```python
from build123d import *

# Parameters (mm, degrees)
BOSS_EXTRUDE1_DEPTH = 6
CHAMFER1_SIZE       = 1
SKETCH2_R           = 1.5
BOSS_EXTRUDE2_DEPTH = 0.7
CHAMFER2_SIZE       = 1
FILLET1_R           = 0.5
BOSS_EXTRUDE3_DEPTH = 1
BOSS_EXTRUDE4_START = 6
BOSS_EXTRUDE4_DEPTH = 1


with BuildPart() as part:
    # Sketch1 → Boss-Extrude1 (new body)
    with BuildSketch(Plane.XY):
        with BuildLine():
            ThreePointArc((0.3, -8), (-0.712809438, -8.999917956), (-1.699671837, -7.974383226))
            Line((-1.699671837, -7.974383226), (-0.822800703, -2.420866047))
            Line((-0.822800703, -2.420866047), (-1.647054908, -1.729905435))
            Line((-1.647054908, -1.729905435), (-1.454328442, -1.5))
            Line((-1.454328442, -1.5), (-0.5, -2.3))
            Line((-0.5, -2.3), (-1.4, -8))
            ThreePointArc((-1.4, -8), (-0.7, -8.7), (0, -8))
            Line((0, -8), (0, 0))
            Line((0, 0), (0.3, 0))
            Line((0.3, 0), (0.3, -8))
        make_face()
    extrude(amount=BOSS_EXTRUDE1_DEPTH)

    # Chamfer1
    chamfer1_edges = [part.edges().sort_by_distance(p)[0] for p in [
        (-1.550691675, -1.614952718, 0),
        (-1.550691675, -1.614952718, 6),
    ]]
    chamfer(chamfer1_edges, length=CHAMFER1_SIZE)

    # Sketch2 → Boss-Extrude2 (add)
    with BuildSketch(Plane(origin=(0.3, 0, 0), x_dir=(0, 0, -1), z_dir=(1, 0, 0))):
        with Locations((-3, -4.3)):
            Circle(SKETCH2_R)
    extrude(amount=BOSS_EXTRUDE2_DEPTH)

    # Chamfer2
    # the kernel refuses this chamfer: 1 mm, written as the material it adds along each edge
    with BuildSketch(Plane(origin=(0.3, -4.3, 3), x_dir=(0, 0, -1), z_dir=(0, -1, 0))) as chamfer2_piece_1_section:
        Polygon((1.5 + CHAMFER2_SIZE, 0), (1.5, CHAMFER2_SIZE), (1.5, 0), align=None)
    chamfer2_piece_1 = revolve(axis=Axis((0.3, -4.3, 3), (1, 0, 0)), mode=Mode.PRIVATE)
    chamfer2_piece_1 = split(chamfer2_piece_1, bisect_by=Plane(origin=(1, -4.3, 5.151462954), z_dir=(-1, 0, 0)), keep=Keep.TOP, mode=Mode.PRIVATE)
    add(chamfer2_piece_1)

    # Fillet1
    fillet1_edges = [part.edges().sort_by_distance(p)[0] for p in [
        (0.3, -4.3, 5.5),
        (1, -4.3, 4.8),
    ]]
    fillet(fillet1_edges, radius=FILLET1_R)

    # Sketch1<3> → Boss-Extrude3 (add)
    with BuildSketch(Plane.XY):
        Polygon((-0.878934414, -4.699917956), (-0.962606384, -5.229840435), (-0.621188888, -5.961100292), (-0.349357155, -5.83418493), align=None)
    extrude(amount=BOSS_EXTRUDE3_DEPTH)

    # Sketch1<4> → Boss-Extrude4 (add)
    with BuildSketch(Plane.XY.offset(BOSS_EXTRUDE4_START)):
        Polygon((-0.878934414, -4.699917956), (-0.962606384, -5.229840435), (-0.621188888, -5.961100292), (-0.349357155, -5.83418493), align=None)
    extrude(amount=-BOSS_EXTRUDE4_DEPTH)


solid = part.part
```
Source: CAD feature listing. Evaluate the final solid. Frame: model axes, mm. A direction names the side the tool comes from. Coordinates: 2 decimals unless noted, no trailing zeros. Write each loop counter-clockwise with the first axis right and the second up, starting at its lowest first coordinate (ties: lowest second). Pieces come first, ordered by that corner, then holes. Notation, with made-up numbers: M 16,-39 L 47,-39 A7 cw 47,-33 Z; hole C 0,31 d1. An arc over 180 degrees is marked long. Answer as a JSON object with one key per item and string values.
1. Access query for faces 1 (the flat face through (0, -4, 3)), 2 (the flat face through (1, -4, 3)), 3 (the flat face through (-0.6, -5.3, 5.5)), 4 (the flat face through (-1.267, -5.236, 2.958)). Directions: +Z, -Z, +X, -X, +Y, -Y. A direction counts if a zero-diameter tool reaches every point of the face in a straight line with its end or side. Return the directions, or none.
Evaluation:
{"face 1": "+Z, -Z, +Y", "face 2": "+Z, -Z, +X, +Y, -Y", "face 3": "+Z, -Z", "face 4": "+Z, -Z, -X"}
2. Cut plane C-C on y = -1.25. Output: boundary loops of the cut face in (x, z).
Evaluation:
{"outline": "M 0,0 L 0.3,0 L 0.3,6 L 0,6 Z"}
3. Cut plane B-B on y = -7.5. Output: boundary loops of the cut face in (x, z).
Evaluation:
{"outline": "M -1.62,0 L -1.32,0 L -1.32,6 L -1.62,6 Z; M 0,0 L 0.3,0 L 0.3,6 L 0,6 Z"}
4. Ray query, L1, parallel to X at y = -5.75, z = 0.75; L2, parallel to X at y = -8, z = 5.75; L3, parallel to X at y = -1.25, z = 4.25. Return the intervals inside material, ascending.
Evaluation:
{"L1": "-1.35 to -1.04, -0.72 to -0.39, 0 to 0.3", "L2": "-1.7 to -1.4, 0 to 0.3", "L3": "0 to 0.3"}
5. Cut plane D-D on x = 0.55. Output: boundary loops of the cut face in (y, z).
Evaluation:
{"outline": "C -4.3,3 d4.5"}
6. Cut plane A-A on z = 3. Output: boundary loops of the cut face in (x, y), plus the area to 3 significant figures.
Evaluation:
{"outline": "M -1.7,-7.97 A1 ccw long 0.3,-8 L 0.3,-7.01 A0.5 cw 0.45,-6.65 L 0.85,-6.25 A0.5 ccw 1,-5.89 L 1,-2.71 A0.5 ccw 0.85,-2.35 L 0.45,-1.95 A0.5 cw 0.3,-1.59 L 0.3,0 L 0,0 L 0,-8 A0.7 cw -1.4,-8 L -0.5,-2.3 L -1.45,-1.5 L -1.65,-1.73 L -0.82,-2.42 Z", "area": "8.27 mm^2"}
7. Draft query along Y for faces 5 (the flat face through (-1.23, -2.08, 2.96)), 6 (the flat face through (0.3, -1, 3)), 7 (the flat face through (-0.984, -1.894, 2.958)). Return one class per face: released by +Y, released by -Y, zero draft, split by the parting line, or undercut.
Evaluation:
{"face 5": "undercut", "face 6": "zero draft", "face 7": "released by +Y"}
